```python
from build123d import *

# Parameters (mm, degrees)
SKETCH2_R               = 33
BOSS_EXTRUDE1_DEPTH     = 8
SKETCH6_R               = 10
BOSS_EXTRUDE2_DEPTH     = 2
CUT_EXTRUDE1_DEPTH      = 48.728398255
CUT_EXTRUDE1_DEPTH_BACK = 48.728398255
SKETCH3_R               = 1.7
SKETCH3_R_2             = 3
CUT_EXTRUDE2_DEPTH      = 48.349762407
CUT_EXTRUDE2_DEPTH_BACK = 2
SKETCH4_R               = 2.8
SKETCH5_R               = 2.1
CUT_EXTRUDE3_DEPTH      = 6
FILLET1_R               = 1
SKETCH7_R               = 11.05
CUT_EXTRUDE4_DEPTH      = 2


with BuildPart() as part:
    # Sketch2 → Boss-Extrude1 (new body)
    with BuildSketch(Plane.XY):
        Circle(SKETCH2_R)
    extrude(amount=BOSS_EXTRUDE1_DEPTH)

    # Sketch6 → Boss-Extrude2 (add)
    with BuildSketch(Plane(origin=(0, 0, 0), x_dir=(-1, 0, 0), z_dir=(0, 0, -1))):
        Circle(SKETCH6_R)
    extrude(amount=BOSS_EXTRUDE2_DEPTH)

    # Sketch3 → Cut-Extrude1 (cut, two sides: drawn at the far end of the back side and taken through both)
    with BuildSketch(Plane.XY.offset(8).offset(-CUT_EXTRUDE1_DEPTH_BACK)):
        with Locations((-15.5, 15.5)):
            Circle(SKETCH3_R)
        with Locations((15.5, 15.5)):
            Circle(SKETCH3_R)
        with Locations((15.5, -15.5)):
            Circle(SKETCH3_R)
        with Locations((-15.5, -15.5)):
            Circle(SKETCH3_R)
        Circle(SKETCH3_R_2)
    extrude(amount=CUT_EXTRUDE1_DEPTH + CUT_EXTRUDE1_DEPTH_BACK, mode=Mode.SUBTRACT)

    # Sketch4 → Cut-Extrude2 (cut, two sides: drawn at the far end of the back side and taken through both)
    with BuildSketch(Plane(origin=(0, 0, 0), x_dir=(-1, 0, 0), z_dir=(0, 0, -1)).offset(-CUT_EXTRUDE2_DEPTH_BACK)):
        with Locations(Location((-15.5, 15.5, 0), (0, 0, 180))):
            Circle(SKETCH4_R)
        with Locations(Location((15.5, 15.5, 0), (0, 0, 180))):
            Circle(SKETCH4_R)
        with Locations(Location((15.5, -15.5, 0), (0, 0, 180))):
            Circle(SKETCH4_R)
        with Locations(Location((-15.5, -15.5, 0), (0, 0, 180))):
            Circle(SKETCH4_R)
    extrude(amount=CUT_EXTRUDE2_DEPTH + CUT_EXTRUDE2_DEPTH_BACK, mode=Mode.SUBTRACT)

    # Sketch5 → Cut-Extrude3 (cut)
    with BuildSketch(Plane(origin=(0, 0, 0), x_dir=(-1, 0, 0), z_dir=(0, 0, -1))):
        with Locations((0, 29.5)):
            Circle(SKETCH5_R)
        with Locations((29.5, 0)):
            Circle(SKETCH5_R)
        with Locations((0, -29.5)):
            Circle(SKETCH5_R)
        with Locations((-29.5, 0)):
            Circle(SKETCH5_R)
    extrude(amount=-CUT_EXTRUDE3_DEPTH, mode=Mode.SUBTRACT)

    # Fillet1
    fillet1_edges = [part.edges().sort_by_distance(p)[0] for p in [
        (10, 0, 0),
    ]]
    fillet(fillet1_edges, radius=FILLET1_R)

    # Sketch7 → Cut-Extrude4 (cut)
    with BuildSketch(Plane.XY.offset(8)):
        Circle(SKETCH7_R)
    extrude(amount=-CUT_EXTRUDE4_DEPTH, mode=Mode.SUBTRACT)


solid = part.part
```
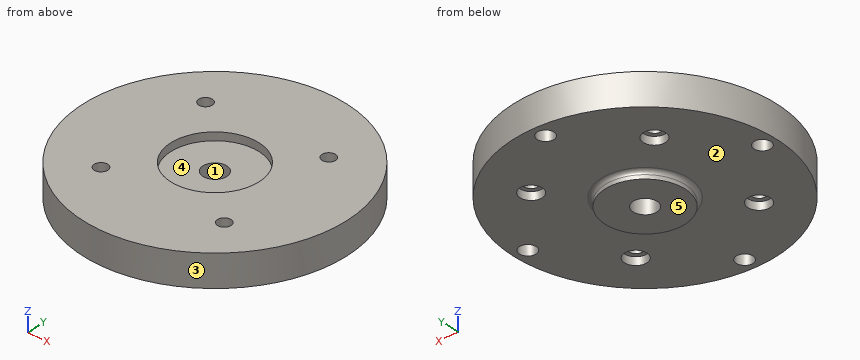
Source: CAD feature listing. Evaluate the final solid. Frame: model axes, mm. Face numbers are marked on the shaded views. A direction names the side the tool comes from. Round coordinates to 2 decimals unless told otherwise and drop trailing zeros. Loops run counter-clockwise (first coordinate to the right, second up) from the corner with the lowest first, then second, coordinate; pieces in that order, holes last. Notation, with made-up numbers: (57, 52.5) - (93, 52.5) arc R16 ccw to (93, 74.5) - close; hole circle Ø7 at (86, 34). An arc over 180 degrees is marked (long way). Use CSV: the item, a comma, the result in double quotes.
Q1. Section query A-A, the plane y = 0. Output: boundary loops of the cut face in (x, z), then the cut area to 3 significant figures.
Reported:
outline,"(-33, 0) - (-31.6, 0) - (-31.6, 6) - (-27.4, 6) - (-27.4, 0) - (-11, 0) arc R1 cw to (-10, -1) - (-10, -2) - (-3, -2) - (-3, 6) - (-11.05, 6) - (-11.05, 8) - (-33, 8) - close; (3, -2) - (10, -2) - (10, -1) arc R1 cw to (11, 0) - (27.4, 0) - (27.4, 6) - (31.6, 6) - (31.6, 0) - (33, 0) - (33, 8) - (11.05, 8) - (11.05, 6) - (3, 6) - close"
area,"426 mm^2"
Q2. Pin query (flat end, axial travel): pin 1 Ø1.5 at (y, z) = (20, 0) entering from +X; pin 2 Ø3 at (x, y) = (-16, 15.5) entering from -Z; pin 3 Ø6 at (y, z) = (5, 5.5) entering from -X. Return the tip coordinate at first contact, or that it passes through.
Reported:
pin 1,"x = 26.8"
pin 2,"z = 2"
pin 3,"x = -32.94"
Q3. Mould query, pull axis Y, two halves, no side actions, for the marked faces 3, 4 and 5. Classes: pulls with the +Y half, pulls with the -Y half, needs draft (parallel to the pull), parting line crosses it, or undercut.
Reported:
face 3,"parting line crosses it"
face 4,"undercut"
face 5,"needs draft"
Q4. Ray query, line 1 along X through (y, z) = (0.5, 7.5); line 2 along X through (y, z) = (15.5, 1.35); line 3 along Y through (x, z) = (15.5, 6). Return the intervals inside material, ascending.
Reported:
line 1,"-33 to -11.04, 11.04 to 33"
line 2,"-29.13 to -18.3, -12.7 to 12.7, 18.3 to 29.13"
line 3,"-29.13 to -17.2, -13.8 to 13.8, 17.2 to 29.13"
Q5. Reachability of the marked faces 1 and 2 from +Z, -Z, +X, -X, +Y, -Y: full face, straight path, thin tool, end or side. Return the list, or none.
Reported:
face 1,"+Z, -Z"
face 2,"-Z"
Q6. Section query B-B, the plane z = 5. Give the number of separate pieces and of enclosed holes in the cut face, then the cut area to 3 significant figures.
Reported:
separate pieces,"1"
enclosed holes,"9"
area,"3,300 mm^2"
Q7. Section query C-C, the plane x = 15.5. Output: boundary loops of the cut face in (y, z).
Reported:
outline,"(-29.13, 0) - (-18.3, 0) - (-18.3, 2) - (-17.2, 2) - (-17.2, 8) - (-29.13, 8) - close; (-13.8, 2) - (-12.7, 2) - (-12.7, 0) - (12.7, 0) - (12.7, 2) - (13.8, 2) - (13.8, 8) - (-13.8, 8) - close; (17.2, 2) - (18.3, 2) - (18.3, 0) - (29.13, 0) - (29.13, 8) - (17.2, 8) - close"
